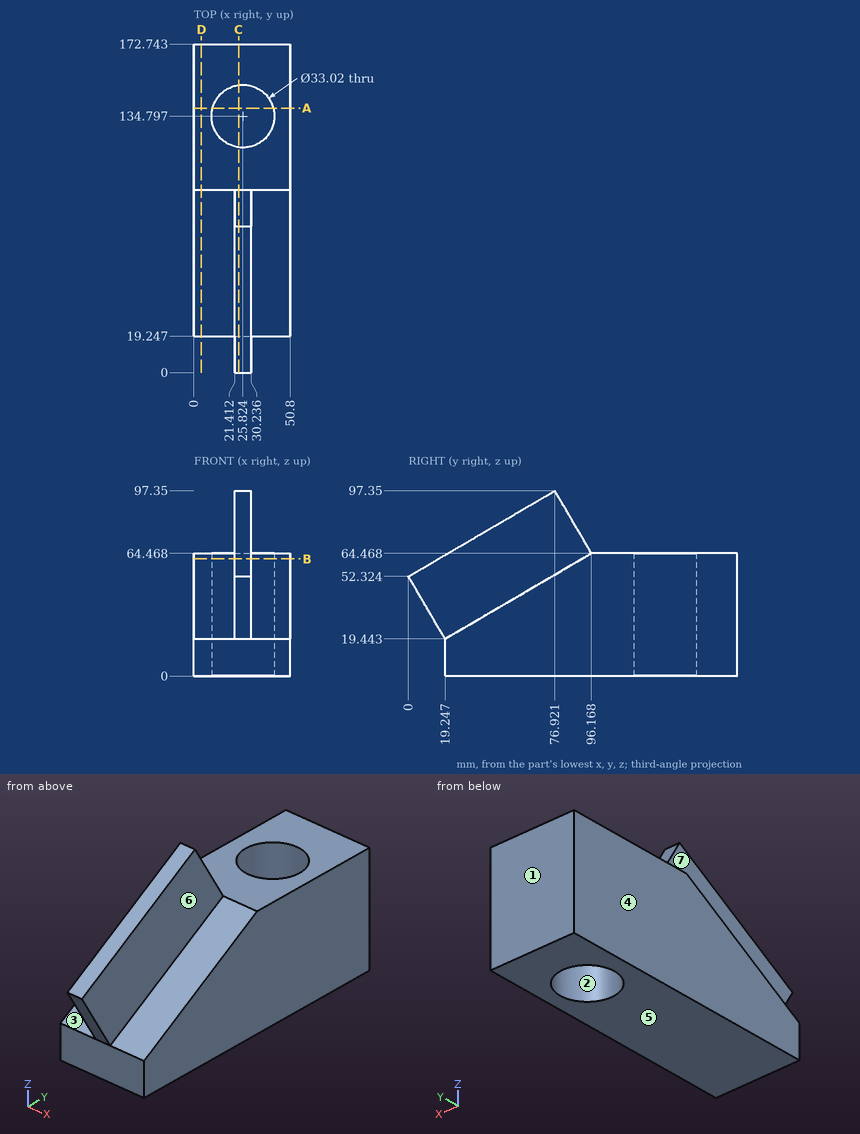
Design review of the part shown in the three views and the two pictorial views. Dimensions are in mm from the part's minimum x, y and z. A direction names the side the tool comes from. Give positions to 0.01 mm unless a question says otherwise; leave off trailing zeros. Order: outer loops, then holes, each group sorted by start corner. A loop starts at its lowest first (then second) coordinate and runs counter-clockwise, first axis right, second up. Notation, with made-up numbers: M 70,4 L 86,4 A24 cw 86,15 Z; hole C 84,27 d11. An arc over 180 degrees is marked long. Answer in a Markdown table with one row per item. Add a question column.
(1) Consider section A-A on y = 139. State the section outline as (x, z) points, and give its area (3 significant figures).
(2) For pin 1 (6 mm diameter, centred on x = 12, y = 76, fed in from +Z); pin 2 (5 mm diameter, centred on y = 88.5, z = 72, fed in from -X); pin 3 (8 mm diameter, centred on x = 25.5, y = 40, fed in from +Z), all flat-tipped, find the tip position at first contact; note any pin that passes through.
(3) For the marked faces 5, 6 and 7, list the 3-axis set-ups (+Z, -Z, +X, -X, +Y, -Y) from which the entire face can be reached by the end or side of a thin tool; tool diameter is ignored.
(4) Consider section C-C on x = 23.5. State the section outline as (y, z) points, and give its area (3 significant figures).
(5) Consider section B-B on z = 61.5. State the section outline as (x, y) points (1 decimal).
(6) Consider section D-D on x = 4. State the section outline as (y, z) points.
(7) Wall thickness on probe 1 along X at (y, z) = (67, 72) (1 decimal); probe 2 along Z at (x, y) = (48.5, 102); probe 3 along X at (y, z) = (149.5, 7) (1 decimal): over which ranges is each line inside the solid? List them lowest first. Write a range as [from, to].
(8) Mouldability with a two-part tool opening along Y and no side actions: class the marked faces 1, 2, 3 and 4 as +Y half, -Y half, draft (parallel to the pull), parting line (faces both ways), or undercut.
Evaluation:
| question | item | result |
|---|---|---|
| 1 | outline | M 0,0 L 9.86,0 L 9.86,64.47 L 0,64.47 Z; M 41.79,0 L 50.8,0 L 50.8,64.47 L 41.79,64.47 Z |
| 1 | area | 1,220 mm^2 |
| 2 | pin 1 | stops at z = 54.42 |
| 2 | pin 2 | stops at x = 21.41 |
| 2 | pin 3 | stops at z = 78.08 |
| 3 | face 5 | -Z, +X, -X, +Y, -Y |
| 3 | face 6 | +Z, +X, -Y |
| 3 | face 7 | +Z, -X, -Y |
| 4 | outline | M 0,52.32 L 19.25,19.44 L 19.25,0 L 118.45,0 L 118.45,64.47 L 96.17,64.47 L 76.92,97.35 Z; M 151.14,0 L 172.74,0 L 172.74,64.47 L 151.14,64.47 Z |
| 4 | area | 9,450 mm^2 |
| 5 | outline | M 0,91.1 L 21.4,91.1 L 21.4,15.7 L 30.2,15.7 L 30.2,91.1 L 50.8,91.1 L 50.8,172.7 L 0,172.7 Z; hole C 25.8,134.8 d33 |
| 6 | outline | M 19.25,0 L 172.74,0 L 172.74,64.47 L 96.17,64.47 L 19.25,19.44 Z |
| 7 | probe 1 | x = [21.4, 30.2] |
| 7 | probe 2 | z = [0, 64.47] |
| 7 | probe 3 | x = [0, 18.3], [33.3, 50.8] |
| 8 | face 1 | +Y half |
| 8 | face 2 | undercut |
| 8 | face 3 | -Y half |
| 8 | face 4 | draft |
